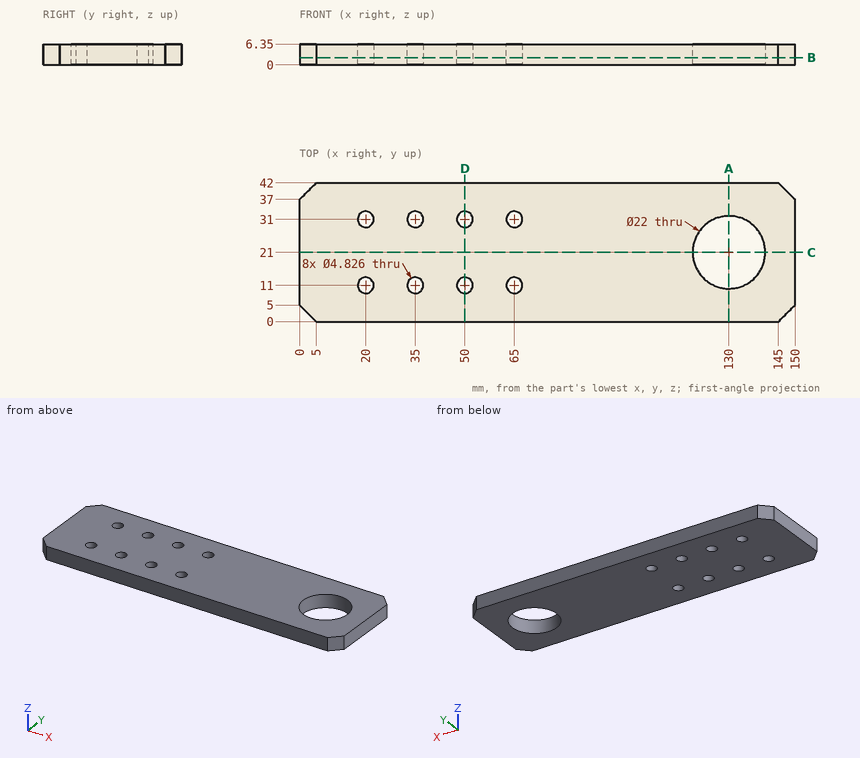
Study the drawing (mm; zero at the part's minimum x, y, z) and answer. Round coordinates to 2 decimals unless told otherwise and drop trailing zeros. Write each loop counter-clockwise with the first axis right and the second up, starting at its lowest first coordinate (ties: lowest second). Pieces come first, ordered by that corner, then holes.
1) A cutting plane is placed at D-D on x = 50. Determine the outline of the cut face in (y, z), and give its area (3 significant figures).
2) A cutting plane is placed at C-C on y = 21. Determine the outline of the cut face in (x, z), and give its area (3 significant figures).
3) A cutting plane is placed at B-B on z = 2.25. Give the number of separate pieces and of enclosed holes in the cut face, and give its area (3 significant figures).
4) Consider probe 1 along Y at (x, z) = (50, 3.5); probe 2 along Y at (x, z) = (130, 3.5); probe 3 along Y at (x, z) = (33.5, 5.75). Determine where each line is inside the solid, lowest interval first.
5) A cutting plane is placed at A-A on x = 130. Determine the outline of the cut face in (y, z), and give its area (3 significant figures).
Entries:
1. outline: (0, 0) - (8.59, 0) - (8.59, 6.35) - (0, 6.35) - close; (13.41, 0) - (28.59, 0) - (28.59, 6.35) - (13.41, 6.35) - close; (33.41, 0) - (42, 0) - (42, 6.35) - (33.41, 6.35) - close
1. area: 205 mm2
2. outline: (0, 0) - (119, 0) - (119, 6.35) - (0, 6.35) - close; (141, 0) - (150, 0) - (150, 6.35) - (141, 6.35) - close
2. area: 813 mm2
3. separate pieces: 1
3. enclosed holes: 9
3. area: 5,720 mm2
4. probe 1: y = 0 to 8.59, 13.41 to 28.59, 33.41 to 42
4. probe 2: y = 0 to 10, 32 to 42
4. probe 3: y = 0 to 9.11, 12.89 to 29.11, 32.89 to 42
5. outline: (0, 0) - (10, 0) - (10, 6.35) - (0, 6.35) - close; (32, 0) - (42, 0) - (42, 6.35) - (32, 6.35) - close
5. area: 127 mm2
